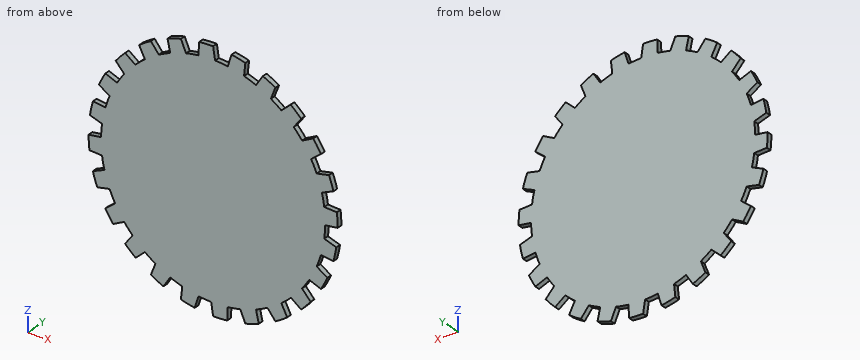
```python
from build123d import *

# Parameters (mm, degrees)
F1_DEPTH = 2


with BuildPart() as f1:
    # F0 (on Front) → F1 (new body)
    with BuildSketch(Plane.XZ):
        with BuildLine():
            Line((-5.660161, 49.678593), (-5.873679, 44.615019))
            ThreePointArc((-5.873679, 44.615019), (-8.393582, 44.210268), (-10.886485, 43.663308))
            Line((-10.886485, 43.663308), (-12.940952, 48.296291))
            ThreePointArc((-12.940952, 48.296291), (-15.65819, 47.484956), (-18.325061, 46.520878))
            Line((-18.325061, 46.520878), (-17.220754, 41.574579))
            ThreePointArc((-17.220754, 41.574579), (-19.550037, 40.531421), (-21.816433, 39.357887))
            Line((-21.816433, 39.357887), (-25, 43.30127))
            ThreePointArc((-25, 43.30127), (-27.414661, 41.814308), (-29.741139, 40.192843))
            Line((-29.741139, 40.192843), (-27.394264, 35.7009))
            ThreePointArc((-27.394264, 35.7009), (-29.374189, 34.090424), (-31.259627, 32.370291))
            Line((-31.259627, 32.370291), (-35.355339, 35.355339))
            ThreePointArc((-35.355339, 35.355339), (-37.302869, 33.294083), (-39.130408, 31.125732))
            Line((-39.130408, 31.125732), (-35.7009, 27.394264))
            ThreePointArc((-35.7009, 27.394264), (-37.196539, 25.326222), (-38.572529, 23.176713))
            Line((-38.572529, 23.176713), (-43.30127, 25))
            ThreePointArc((-43.30127, 25), (-44.648947, 22.504922), (-45.853004, 19.937453))
            Line((-45.853004, 19.937453), (-41.574579, 17.220754))
            ThreePointArc((-41.574579, 17.220754), (-42.484006, 14.836079), (-43.256776, 12.403681))
            Line((-43.256776, 12.403681), (-48.296291, 12.940952))
            ThreePointArc((-48.296291, 12.940952), (-48.952274, 10.182088), (-49.450793, 7.390471))
            Line((-49.450793, 7.390471), (-44.615019, 5.873679))
            ThreePointArc((-44.615019, 5.873679), (-44.876258, 3.334882), (-44.993146, 0.785358))
            Line((-44.993146, 0.785358), (-50, 0))
            ThreePointArc((-50, 0), (-49.919584, -2.834639), (-49.678593, -5.660161))
            Line((-49.678593, -5.660161), (-44.615019, -5.873679))
            ThreePointArc((-44.615019, -5.873679), (-44.210268, -8.393582), (-43.663308, -10.886485))
            Line((-43.663308, -10.886485), (-48.296291, -12.940952))
            ThreePointArc((-48.296291, -12.940952), (-47.484956, -15.65819), (-46.520878, -18.325061))
            Line((-46.520878, -18.325061), (-41.574579, -17.220754))
            ThreePointArc((-41.574579, -17.220754), (-40.531421, -19.550037), (-39.357887, -21.816433))
            Line((-39.357887, -21.816433), (-43.30127, -25))
            ThreePointArc((-43.30127, -25), (-41.814308, -27.414661), (-40.192843, -29.741139))
            Line((-40.192843, -29.741139), (-35.7009, -27.394264))
            ThreePointArc((-35.7009, -27.394264), (-34.090424, -29.374189), (-32.370291, -31.259627))
            Line((-32.370291, -31.259627), (-35.355339, -35.355339))
            ThreePointArc((-35.355339, -35.355339), (-33.294083, -37.302869), (-31.125732, -39.130408))
            Line((-31.125732, -39.130408), (-27.394264, -35.7009))
            ThreePointArc((-27.394264, -35.7009), (-25.326222, -37.196539), (-23.176713, -38.572529))
            Line((-23.176713, -38.572529), (-25, -43.30127))
            ThreePointArc((-25, -43.30127), (-22.504922, -44.648947), (-19.937453, -45.853004))
            Line((-19.937453, -45.853004), (-17.220754, -41.574579))
            ThreePointArc((-17.220754, -41.574579), (-14.836079, -42.484006), (-12.403681, -43.256776))
            Line((-12.403681, -43.256776), (-12.940952, -48.296291))
            ThreePointArc((-12.940952, -48.296291), (-10.182088, -48.952274), (-7.390471, -49.450793))
            Line((-7.390471, -49.450793), (-5.873679, -44.615019))
            ThreePointArc((-5.873679, -44.615019), (-3.334882, -44.876258), (-0.785358, -44.993146))
            Line((-0.785358, -44.993146), (0, -50))
            ThreePointArc((0, -50), (2.834639, -49.919584), (5.660161, -49.678593))
            Line((5.660161, -49.678593), (5.873679, -44.615019))
            ThreePointArc((5.873679, -44.615019), (8.393582, -44.210268), (10.886485, -43.663308))
            Line((10.886485, -43.663308), (12.940952, -48.296291))
            ThreePointArc((12.940952, -48.296291), (15.65819, -47.484956), (18.325061, -46.520878))
            Line((18.325061, -46.520878), (17.220754, -41.574579))
            ThreePointArc((17.220754, -41.574579), (19.550037, -40.531421), (21.816433, -39.357887))
            Line((21.816433, -39.357887), (25, -43.30127))
            ThreePointArc((25, -43.30127), (27.414661, -41.814308), (29.741139, -40.192843))
            Line((29.741139, -40.192843), (27.394264, -35.7009))
            ThreePointArc((27.394264, -35.7009), (29.374189, -34.090424), (31.259627, -32.370291))
            Line((31.259627, -32.370291), (35.355339, -35.355339))
            ThreePointArc((35.355339, -35.355339), (37.302869, -33.294083), (39.130408, -31.125732))
            Line((39.130408, -31.125732), (35.7009, -27.394264))
            ThreePointArc((35.7009, -27.394264), (37.196539, -25.326222), (38.572529, -23.176713))
            Line((38.572529, -23.176713), (43.30127, -25))
            ThreePointArc((43.30127, -25), (44.648947, -22.504922), (45.853004, -19.937453))
            Line((45.853004, -19.937453), (41.574579, -17.220754))
            ThreePointArc((41.574579, -17.220754), (42.484006, -14.836079), (43.256776, -12.403681))
            Line((43.256776, -12.403681), (48.296291, -12.940952))
            ThreePointArc((48.296291, -12.940952), (48.952274, -10.182088), (49.450793, -7.390471))
            Line((49.450793, -7.390471), (44.615019, -5.873679))
            ThreePointArc((44.615019, -5.873679), (44.876258, -3.334882), (44.993146, -0.785358))
            Line((44.993146, -0.785358), (50, 0))
            ThreePointArc((50, 0), (49.919584, 2.834639), (49.678593, 5.660161))
            Line((49.678593, 5.660161), (44.615019, 5.873679))
            ThreePointArc((44.615019, 5.873679), (44.210268, 8.393582), (43.663308, 10.886485))
            Line((43.663308, 10.886485), (48.296291, 12.940952))
            ThreePointArc((48.296291, 12.940952), (47.484956, 15.65819), (46.520878, 18.325061))
            Line((46.520878, 18.325061), (41.574579, 17.220754))
            ThreePointArc((41.574579, 17.220754), (40.531421, 19.550037), (39.357887, 21.816433))
            Line((39.357887, 21.816433), (43.30127, 25))
            ThreePointArc((43.30127, 25), (41.814308, 27.414661), (40.192843, 29.741139))
            Line((40.192843, 29.741139), (35.7009, 27.394264))
            ThreePointArc((35.7009, 27.394264), (34.090424, 29.374189), (32.370291, 31.259627))
            Line((32.370291, 31.259627), (35.355339, 35.355339))
            ThreePointArc((35.355339, 35.355339), (33.294083, 37.302869), (31.125732, 39.130408))
            Line((31.125732, 39.130408), (27.394264, 35.7009))
            ThreePointArc((27.394264, 35.7009), (25.326222, 37.196539), (23.176713, 38.572529))
            Line((23.176713, 38.572529), (25, 43.30127))
            ThreePointArc((25, 43.30127), (22.504922, 44.648947), (19.937453, 45.853004))
            Line((19.937453, 45.853004), (17.220754, 41.574579))
            ThreePointArc((17.220754, 41.574579), (14.836079, 42.484006), (12.403681, 43.256776))
            Line((12.403681, 43.256776), (12.940952, 48.296291))
            ThreePointArc((12.940952, 48.296291), (10.182088, 48.952274), (7.390471, 49.450793))
            Line((7.390471, 49.450793), (5.873679, 44.615019))
            ThreePointArc((5.873679, 44.615019), (3.334882, 44.876258), (0.785358, 44.993146))
            Line((0.785358, 44.993146), (0, 50))
            ThreePointArc((0, 50), (-2.834639, 49.919584), (-5.660161, 49.678593))
        make_face()
    extrude(amount=F1_DEPTH)


solid = f1.part
```
For this review, take the finished solid that the model builds, in its own axes (mm). Round coordinates to 2 decimals unless told otherwise and drop trailing zeros. Loops run counter-clockwise (first coordinate to the right, second up) from the corner with the lowest first, then second, coordinate; pieces in that order, holes last.
Q1. Add section B-B on z = -15. Write out the cut boundary in (x, y), plus the area to 3 significant figures.
Result sheet:
outline: (-47.7, -2) - (42.43, -2) - (42.43, 0) - (-47.7, 0) - close
area: 180 mm2
Q2. Insertion check: pin 1 Ø1 at (x, y) = (23, 0) entering from +Z. The pin has a flat end and moves straight along its axis. Give the tip position at first contact, or say it passes through.
Result sheet:
pin 1: stops at z = 44.65
Q3. Add section A-A on x = 2. Write out the cut boundary in (y, z), plus the area to 3 significant figures.
Result sheet:
outline: (-2, -49.96) - (0, -49.96) - (0, 44.96) - (-2, 44.96) - close
area: 190 mm2
Q4. To check wall thickness, follow line 1 along Z through (x, y) = (-1, -1.2); line 2 along Z through (x, y) = (-40.5, -0.55); line 3 along Z through (x, y) = (-17, -1.5). State the ranges of each line that lie inside material, in increasing order.
Result sheet:
line 1: z = -44.99 to 49.99
line 2: z = -29.32 to -22.74, -19.62 to 23.92
line 3: z = -41.67 to 47.02
